Here's how the part is built. I have some questions about the finished solid (model axes, mm). A direction names the side the tool comes from. Coordinates: 2 decimals unless noted, no trailing zeros. Loops run counter-clockwise (first coordinate to the right, second up) from the corner with the lowest first, then second, coordinate; pieces in that order, holes last. Notation, with made-up numbers: (14.25, 49) - (72.25, 49) arc R22 cw to (72.25, 87) - close; hole circle Ø5 at (26.25, 81). An arc over 180 degrees is marked (long way). Use a Markdown table: item, result.
```python
from build123d import *

# Parameters (mm, degrees)
F0_W     = 120
F0_H     = 120
F1_DEPTH = 25
F2_R     = 25
F3_DEPTH = 10
F5_D     = 5


with BuildPart() as f1:
    # F0 (on Front) → F1 (new body, symmetric)
    with BuildSketch(Plane.XZ):
        Rectangle(F0_W, F0_H)
    extrude(amount=F1_DEPTH, both=True)

    # F2 (on face) → F3 (cut)
    with BuildSketch(Plane.XZ.offset(25)):
        Circle(F2_R)
    extrude(amount=-F3_DEPTH, mode=Mode.SUBTRACT)

    # F5 (through all)
    with Locations(Plane.XZ.offset(15)):
        with Locations((0, 0)):
            Hole(F5_D / 2)


solid = f1.part
```
Q1. If we mould it in two halves opening along X, with no side actions, what happens to faces 3 (the face through (-60, 0, -1)), 4 (the face through (0, -15, -5)), 5 (the face through (-1, 0, -60)), 6 (the face through (60, 0, -1))? For each: pulls with the +X half, pulls with the -X half, needs draft (parallel to the pull), parting line crosses it, or undercut.
Check values:
| item | result |
|---|---|
| face 3 | pulls with the -X half |
| face 4 | undercut |
| face 5 | needs draft |
| face 6 | pulls with the +X half |
Q2. I want a section at C-C, the plane z = -20. Write out the boundary of the cut face in (x, y), then the cut area to 3 significant figures.
Check values:
| item | result |
|---|---|
| outline | (-60, -25) - (-15, -25) - (-15, -15) - (15, -15) - (15, -25) - (60, -25) - (60, 25) - (-60, 25) - close |
| area | 5,700 mm^2 |
Q3. I want a section at A-A, the plane x = 0. Write out the boundary of the cut face in (y, z).
Check values:
| item | result |
|---|---|
| outline | (-25, -60) - (25, -60) - (25, -2.5) - (-15, -2.5) - (-15, -25) - (-25, -25) - close; (-25, 25) - (-15, 25) - (-15, 2.5) - (25, 2.5) - (25, 60) - (-25, 60) - close |
Q4. I want a section at D-D, the plane x = 23. Write out the boundary of the cut face in (y, z).
Check values:
| item | result |
|---|---|
| outline | (-25, -60) - (25, -60) - (25, 60) - (-25, 60) - (-25, 9.8) - (-15, 9.8) - (-15, -9.8) - (-25, -9.8) - close |
Q5. Which directions (+Z, -Z, +X, -X, +Y, -Y) give clear straight access to the entire face, cutting with the end or side of a thin tool? Please do faces 1 (the face through (23.846, -20.07, 7.509)), 2 (the face through (-1, 0, 60)).
Check values:
| item | result |
|---|---|
| face 1 | -Y |
| face 2 | +Z, +X, -X, +Y, -Y |
Q6. Please list where these lines run through material, in increasing order: L1, parallel to Z at x = 0, y = -3; L2, parallel to Z at x = 0, y = -18.75; L3, parallel to X at y = -20, z = -11.5. Write a range as from..to.
Check values:
| item | result |
|---|---|
| L1 | -60..-2.5, 2.5..60 |
| L2 | -60..-25, 25..60 |
| L3 | -60..-22.2, 22.2..60 |
Q7. I want a section at B-B, the plane z = 0. Write out the boundary of the cut face in (x, y), then the cut area to 3 significant figures.
Check values:
| item | result |
|---|---|
| outline | (-60, -25) - (-25, -25) - (-25, -15) - (-2.5, -15) - (-2.5, 25) - (-60, 25) - close; (2.5, -15) - (25, -15) - (25, -25) - (60, -25) - (60, 25) - (2.5, 25) - close |
| area | 5,300 mm^2 |
Q8. Will this pin go through, and if not, where does the flat tip stop? P1, Ø6.5, axis at x = 0, z = 0, coming from the -Y side.
Check values:
| item | result |
|---|---|
| P1 | y = -15 |
